Geometry check sheet. Reference: drawing and pictorial views, mm from the part's lowest x, y, z. Coordinates: 2 decimals unless noted, no trailing zeros. Loops run counter-clockwise (first coordinate to the right, second up) from the corner with the lowest first, then second, coordinate; pieces in that order, holes last. Notation, with made-up numbers: (-22, 47.25) -> (14, 47.25) arc R26 cw to (14, 66.25) -> close; hole circle Ø3 at (-21, -3). An arc over 180 degrees is marked (long way). Answer as a JSON object with one key per item and string values.
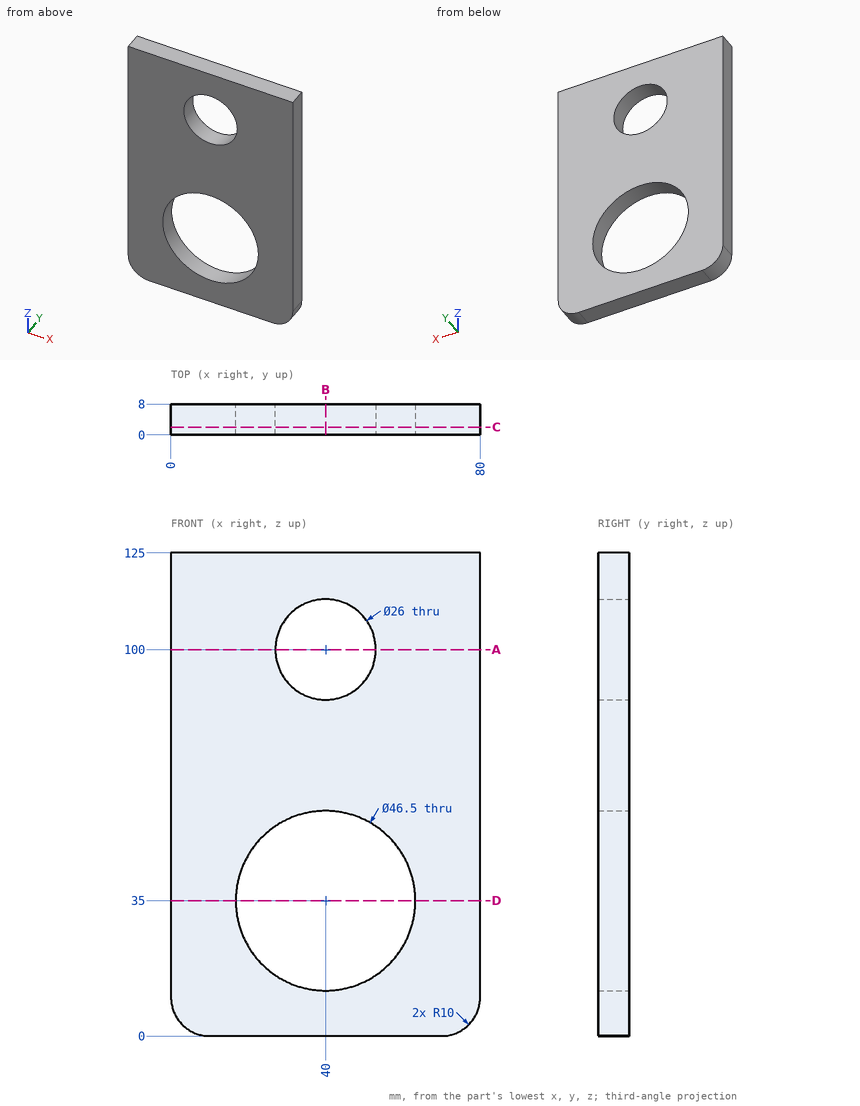
1. Section check B-B, the plane x = 40. Record the boundary of the cut face in (y, z), then the cut area to 3 significant figures.
Evaluation:
{"outline": "(0, 0) -> (8, 0) -> (8, 11.75) -> (0, 11.75) -> close; (0, 58.25) -> (8, 58.25) -> (8, 87) -> (0, 87) -> close; (0, 113) -> (8, 113) -> (8, 125) -> (0, 125) -> close", "area": "420 mm^2"}
2. Section check C-C, the plane y = 2. Record the boundary of the cut face in (x, z), then the cut area to 3 significant figures.
Evaluation:
{"outline": "(0, 10) arc R10 ccw to (10, 0) -> (70, 0) arc R10 ccw to (80, 10) -> (80, 125) -> (0, 125) -> close; hole circle Ø46.5 at (40, 35); hole circle Ø26 at (40, 100)", "area": "7,730 mm^2"}
3. Thickness scan on probe 1 along Z at (x, y) = (40, 5); probe 2 along Z at (x, y) = (36.5, 7); probe 3 along X at (y, z) = (2.25, 101.5). Record the ranges inside material, lowest first. Write a range as from..to.
Evaluation:
{"probe 1": "z = 0..11.75, 58.25..87, 113..125", "probe 2": "z = 0..12.01, 57.99..87.48, 112.52..125", "probe 3": "x = 0..27.09, 52.91..80"}
4. Section check A-A, the plane z = 100. Record the boundary of the cut face in (x, y), then the cut area to 3 significant figures.
Evaluation:
{"outline": "(0, 0) -> (27, 0) -> (27, 8) -> (0, 8) -> close; (53, 0) -> (80, 0) -> (80, 8) -> (53, 8) -> close", "area": "432 mm^2"}
5. Section check D-D, the plane z = 35. Record the boundary of the cut face in (x, y), then the cut area to 3 significant figures.
Evaluation:
{"outline": "(0, 0) -> (16.75, 0) -> (16.75, 8) -> (0, 8) -> close; (63.25, 0) -> (80, 0) -> (80, 8) -> (63.25, 8) -> close", "area": "268 mm^2"}
